```python
from build123d import *

# Parameters (mm, degrees)
CROQUIS1_R              = 15
CROQUIS1_R_2            = 12
EXTRUIR_L_MINA1_DEPTH   = 6.5
CROQUIS2_R              = 5
SALIENTE_EXTRUIR1_DEPTH = 6.5
CROQUIS3_R              = 12.5
SALIENTE_EXTRUIR2_DEPTH = 1
CROQUIS4_R              = 2
SALIENTE_EXTRUIR3_DEPTH = 11
SALIENTE_EXTRUIR4_DEPTH = 22
CROQUIS7_W              = 45
CROQUIS7_H              = 30
CROQUIS7_R              = 2
SALIENTE_EXTRUIR5_DEPTH = 1


with BuildPart() as part:
    # Croquis1 → Extruir-Lámina1 (new, symmetric)
    with BuildSketch(Plane.XY):
        Circle(CROQUIS1_R)
        Circle(CROQUIS1_R_2, mode=Mode.SUBTRACT)
    extrude(amount=EXTRUIR_L_MINA1_DEPTH, both=True)



with BuildPart() as body_2:
    # Croquis2 → Saliente-Extruir1 (new, symmetric)
    with BuildSketch(Plane.XY):
        with Locations(Location((0, 0, 0), (0, 0, 180))):
            Circle(CROQUIS2_R)
    extrude(amount=SALIENTE_EXTRUIR1_DEPTH, both=True)


with BuildPart() as part_1:
    add(part.part)

    add(body_2.part)  # Saliente-Extruir2 merges body 2
    # Croquis3 → Saliente-Extruir2 (add, symmetric)
    with BuildSketch(Plane.XY):
        Circle(CROQUIS3_R)
    extrude(amount=SALIENTE_EXTRUIR2_DEPTH, both=True)

    # Croquis4 → Saliente-Extruir3 (add, symmetric)
    with BuildSketch(Plane.XY):
        Circle(CROQUIS4_R)
    extrude(amount=SALIENTE_EXTRUIR3_DEPTH, both=True)

    # Croquis6 → Saliente-Extruir4 (add, through all)
    with BuildSketch(Plane.XY.offset(11)):
        with BuildLine():
            Line((-4.581858608, 2.977952867), (7.949667258, 22))
            Line((7.949667258, 22), (27.086339579, 22))
            Line((27.086339579, 22), (10.776903307, -2.756671198))
            Line((10.776903307, -2.756671198), (-1.492562871, -2.756671198))
            ThreePointArc((-1.492562871, -2.756671198), (-4.749465591, -0.811766904), (-4.581858608, 2.977952867))
        make_face()
    extrude(amount=-SALIENTE_EXTRUIR4_DEPTH)

    # Croquis7 → Saliente-Extruir5 (add)
    with BuildSketch(Plane(origin=(0, 22, 0), x_dir=(1, 0, 0), z_dir=(0, 1, 0))):
        with Locations((17.519667258, 0)):
            Rectangle(CROQUIS7_W, CROQUIS7_H)
        with Locations(Location((33.519667258, 10, 0), (0, 0, 270))):
            Circle(CROQUIS7_R, mode=Mode.SUBTRACT)
        with Locations(Location((1.519667258, 10, 0), (0, 0, 90))):
            Circle(CROQUIS7_R, mode=Mode.SUBTRACT)
        with Locations(Location((33.519667258, -10, 0), (0, 0, 90))):
            Circle(CROQUIS7_R, mode=Mode.SUBTRACT)
        with Locations(Location((1.519667258, -10, 0), (0, 0, 270))):
            Circle(CROQUIS7_R, mode=Mode.SUBTRACT)
    extrude(amount=-SALIENTE_EXTRUIR5_DEPTH)


solid = part_1.part
```
Model file for the job. Use its own axes, mm. A direction names the side the tool comes from. Coordinates: 2 decimals unless noted, no trailing zeros. Loops run counter-clockwise (first coordinate to the right, second up) from the corner with the lowest first, then second, coordinate; pieces in that order, holes last. Notation, with made-up numbers: (74, 10) - (83, 10) arc R19 cw to (83, 45) - close; hole circle Ø7 at (21, 67.25). An arc over 180 degrees is marked (long way). Answer as a JSON object with one key per item and string values. Group by question number.
(1) Cut at D-D (z = 0.25). Give the cut face in (x, y), then the cut area to 3 significant figures.
(2) Flat gauge pins, fed straight in: pin 1 (4 mm diameter, centred on x = 1, y = -1.5, fed in from +Z); pin 2 (4 mm diameter, centred on x = -1, y = -2, fed in from -Z); pin 3 (6 mm diameter, centred on y = -4, z = -5.5, fed in from -X). Where does each tip first touch, or does it go through?
(3) Two-plate mould, pull along Z, no slides. Class faces 1 (the face through (2.737, 21.507, -8.413)), 2 (the face through (31.567, 21.507, -10.434)), 3 (the face through (0, -4, 6.5)), 4 (the face through (-11, -10.2, 0.1)): released by +Z, released by -Z, zero draft, split by the parting line, or undercut.
(4) Probe line 1 along X through (y, z) = (21.6, -10); line 2 along Y through (x, z) = (0, -3.6); line 3 along Y through (x, z) = (34.5, 4.75). List the from-to ranges inside material, lowest first.
(5) Cut at A-A (z = 10). Give the cut face in (x, y), then the cut area to 3 significant figures.
(6) Tool access for faces 5 (the face through (11, 9, 11)), 6 (the face through (-5.06, -0.04, 7.18)), 7 (the face through (11, 9, -11)), 8 (the face through (31.537, 21.507, 10.26)), 9 (the face through (-5.06, -0.04, -7.04)): list every direction of +Z, -Z, +X, -X, +Y, -Y with a clear straight run to the whole face (end or side of a thin tool).
(7) Cut at C-C (x = 19). Give the cut face in (y, z).
(8) Cut at B-B (z = 5.5). Give the cut face in (x, y), then the cut area to 3 significant figures.
Geometry says:
{
 "1": {"outline": "(-4.98, 21) - (7.29, 21) - (3.12, 14.67) arc R15 ccw (long way) to (14.67, 3.15) - (26.43, 21) - (40.02, 21) - (40.02, 22) - (-4.98, 22) - close", "area": "957 mm^2"},
 "2": {"pin 1": "stops at z = 11", "pin 2": "stops at z = -11", "pin 3": "stops at x = -14.97"},
 "3": {"face 1": "undercut", "face 2": "undercut", "face 3": "released by +Z", "face 4": "zero draft"},
 "4": {"line 1": "x = -4.98 to -0.48, 3.52 to 31.52, 35.52 to 40.02", "line 2": "y = -15 to -12, -5 to 9.93, 12 to 15, 21 to 22", "line 3": "y = 21 to 22"},
 "5": {"outline": "(-4.98, 21) - (-0.48, 21) - (-0.48, 22) - (-4.98, 22) - close; (-4.58, 2.98) arc R3.7 ccw to (-1.49, -2.76) - (10.78, -2.76) - (26.43, 21) - (31.52, 21) - (31.52, 22) - (3.52, 22) - (3.52, 21) - (7.29, 21) - close; (35.52, 21) - (40.02, 21) - (40.02, 22) - (35.52, 22) - close", "area": "481 mm^2"},
 "6": {"face 5": "+Z, +X, -X, -Y", "face 6": "+Z", "face 7": "-Z, +X, -X, -Y", "face 8": "+Y, -Y", "face 9": "-Z"},
 "7": {"outline": "(9.73, -11) - (21, -11) - (21, -15) - (22, -15) - (22, 15) - (21, 15) - (21, 11) - (9.73, 11) - close"},
 "8": {"outline": "(-4.98, 21) - (7.29, 21) - (3.12, 14.67) arc R15 ccw (long way) to (14.67, 3.15) - (26.43, 21) - (40.02, 21) - (40.02, 22) - (-4.98, 22) - close; hole (-4.99, -0.25) arc R3.7 cw to (-4.58, 2.98) - (1.31, 11.93) arc R12 ccw (long way) to (11.96, -0.96) - (10.78, -2.76) - (4.17, -2.76) arc R5 cw to start", "area": "705 mm^2"}
}
